from build123d import *

# Parameters (mm, degrees)
F0_W     = 20
F0_H     = 40
F0_W_2   = 1
F0_H_2   = 5
F1_DEPTH = 3.175
F2_DEPTH = 40
F4_D     = 4.0894


# Not quite as in the source:
# - a length typed as a fraction of an inch, garbled in the dataset ("3 / 203.2 mm" for 3/8 in), is restored


with BuildPart() as f1:
    # F0 (on Top) → F1 (new body)
    with BuildSketch(Plane.XY):
        Rectangle(F0_W, F0_H)
        with Locations((-5.5, 7.5)):
            Rectangle(F0_W_2, F0_H_2, mode=Mode.SUBTRACT)
        with Locations((5.5, 7.5)):
            Rectangle(F0_W_2, F0_H_2, mode=Mode.SUBTRACT)
    extrude(amount=F1_DEPTH)

    # F0 (on Top) → F2 (join)
    with BuildSketch(Plane.XY):
        with Locations((-5.5, 7.5)):
            Rectangle(F0_W_2, F0_H_2)
        with Locations((5.5, 7.5)):
            Rectangle(F0_W_2, F0_H_2)
    extrude(amount=F2_DEPTH)

    # F4 (through all)
    with Locations(Plane.YZ.offset(6)):
        with Locations((7.5, 22.175)):
            Hole(F4_D / 2)


solid = f1.part
For this review, take the finished solid that the model builds, in its own axes (mm). A direction names the side the tool comes from. Round coordinates to 2 decimals unless told otherwise and drop trailing zeros. Loops run counter-clockwise (first coordinate to the right, second up) from the corner with the lowest first, then second, coordinate; pieces in that order, holes last. Notation, with made-up numbers: (-13, -31.5) - (35, -31.5) arc R23 cw to (35, -15.5) - close; hole circle Ø7 at (82, -29). An arc over 180 degrees is marked (long way). Answer as CSV lines item,"result".
(1) Consider section C-C on z = 21.5. Give the boundary of the cut face in (x, y), then the cut area to 3 significant figures.
Checked values:
outline,"(-6, 5) - (-5, 5) - (-5, 5.57) - (-6, 5.57) - close; (-6, 9.43) - (-5, 9.43) - (-5, 10) - (-6, 10) - close; (5, 5) - (6, 5) - (6, 5.57) - (5, 5.57) - close; (5, 9.43) - (6, 9.43) - (6, 10) - (5, 10) - close"
area,"2.28 mm2"
(2) Wall thickness on line 1 (X direction, y = 6.5, z = 11.5); line 2 (Z direction, x = -5.7, y = 7.5); line 3 (Z direction, x = -5, y = 17) (3 decimals): over which ranges is each line inside the solid? List them lowest first.
Checked values:
line 1,"x = -6 to -5, 5 to 6"
line 2,"z = 0 to 20.13, 24.22 to 40"
line 3,"z = 0 to 3.175"
(3) Mouldability with a two-part tool opening along X and no side actions: class faces 1 (the face through (-5.5, 7.5, 40)), 2 (the face through (-10, 0, 2)), 3 (the face through (-5, 9.7, 21.3)) as +X half, -X half, draft (parallel to the pull), parting line (faces both ways), or undercut.
Checked values:
face 1,"draft"
face 2,"-X half"
face 3,"undercut"
(4) Consider section A-A on y = 7.5. Give the boundary of the cut face in (x, z) (3 decimals).
Checked values:
outline,"(-10, 0) - (10, 0) - (10, 3.175) - (6, 3.175) - (6, 20.13) - (5, 20.13) - (5, 3.175) - (-5, 3.175) - (-5, 20.13) - (-6, 20.13) - (-6, 3.175) - (-10, 3.175) - close; (-6, 24.22) - (-5, 24.22) - (-5, 40) - (-6, 40) - close; (5, 24.22) - (6, 24.22) - (6, 40) - (5, 40) - close"
(5) Consider section D-D on x = -1.5. Give the boundary of the cut face in (y, z) (3 decimals), then the cut area to 3 significant figures.
Checked values:
outline,"(-20, 0) - (20, 0) - (20, 3.175) - (-20, 3.175) - close"
area,"127 mm2"
(6) Tool access review of faces 4 (the face through (-6, 9.7, 21.3)), 5 (the face through (5, 9.7, 21.3)), 6 (the face through (-5.5, 5, 21.3)), 7 (the face through (5.5, 10, 21.3)): name each direction out of +Z, -Z, +X, -X, +Y, -Y from which nothing blocks a thin tool from reaching the whole face with its end or side.
Checked values:
face 4,"+Z, -X, +Y, -Y"
face 5,"+Z, +Y, -Y"
face 6,"+Z, +X, -X, -Y"
face 7,"+Z, +X, -X, +Y"
(7) Consider section B-B on z = 17.5. Give the boundary of the cut face in (x, y), then the cut area to 3 significant figures.
Checked values:
outline,"(-6, 5) - (-5, 5) - (-5, 10) - (-6, 10) - close; (5, 5) - (6, 5) - (6, 10) - (5, 10) - close"
area,"10.0 mm2"
(8) Insertion check: P1, Ø1.1, axis at x = 5.5, z = 12.5, coming from the -Y side; P2, Ø1.1, axis at x = -5.5, z = 30, coming from the +Y side; P3, Ø6.5, axis at y = 7.5, z = 22.175, coming from the -X side. Each pin has a flat end and moves straight along its axis. Give the tip position at first contact, or say it passes through.
Checked values:
P1,"stops at y = 5"
P2,"stops at y = 10"
P3,"stops at x = -6"
